```python
from build123d import *

# Parameters (mm, degrees)
F0_W      = 1397
F0_H      = 355.6
F1_DEPTH  = 920.75
F9_W      = 330.2
F9_H      = 330.2
F10_DEPTH = 279.4
F7_W      = 330.2
F7_H      = 330.2
F11_DEPTH = 279.4
F5_W      = 330.2
F5_H      = 330.2
F12_DEPTH = 279.4
F3_W      = 330.2
F3_H      = 330.2
F13_DEPTH = 279.4


with BuildPart() as f1:
    # F0 (on Top) → F1 (new body)
    with BuildSketch(Plane.XY):
        with Locations((698.5, -177.8)):
            Rectangle(F0_W, F0_H)
    extrude(amount=F1_DEPTH)

    # F9 (on face) → F10 (cut)
    with BuildSketch(Plane.XY.offset(920.75)):
        with Locations((190.5, -177.8)):
            Rectangle(F9_W, F9_H)
    extrude(amount=-F10_DEPTH, mode=Mode.SUBTRACT)

    # F7 (on face) → F11 (cut)
    with BuildSketch(Plane.XY.offset(920.75)):
        with Locations((533.4, -177.8)):
            Rectangle(F7_W, F7_H)
    extrude(amount=-F11_DEPTH, mode=Mode.SUBTRACT)

    # F5 (on face) → F12 (cut)
    with BuildSketch(Plane.XY.offset(920.75)):
        with Locations((876.3, -177.8)):
            Rectangle(F5_W, F5_H)
    extrude(amount=-F12_DEPTH, mode=Mode.SUBTRACT)

    # F3 (on face) → F13 (cut)
    with BuildSketch(Plane.XY.offset(920.75)):
        with Locations((1219.2, -177.8)):
            Rectangle(F3_W, F3_H)
    extrude(amount=-F13_DEPTH, mode=Mode.SUBTRACT)

    # F14: F1 across plane


with BuildPart() as f1_1:
    add(f1.part)
    add(f1.part.mirror(Plane.XZ))


solid = f1_1.part
```
Source: CAD feature listing. Evaluate the final solid. Frame: model axes, mm. Round coordinates to 2 decimals unless told otherwise and drop trailing zeros. Loops run counter-clockwise (first coordinate to the right, second up) from the corner with the lowest first, then second, coordinate; pieces in that order, holes last. Notation, with made-up numbers: (-35.75, 28) - (15.25, 28) arc R7 ccw to (15.25, 35) - close; hole circle Ø11 at (21, 53). An arc over 180 degrees is marked (long way). Use CSV: the item, a comma, the result in double quotes.
Q1. Section query B-B, the plane y = 253.5. Output: boundary loops of the cut face in (x, z), then the cut area to 3 significant figures.
Reported:
outline,"(0, 0) - (1397, 0) - (1397, 920.75) - (1384.3, 920.75) - (1384.3, 641.35) - (1054.1, 641.35) - (1054.1, 920.75) - (1041.4, 920.75) - (1041.4, 641.35) - (711.2, 641.35) - (711.2, 920.75) - (698.5, 920.75) - (698.5, 641.35) - (368.3, 641.35) - (368.3, 920.75) - (355.6, 920.75) - (355.6, 641.35) - (25.4, 641.35) - (25.4, 920.75) - (0, 920.75) - close"
area,"917,000 mm^2"
Q2. Mould query, pull axis X, two halves, no side actions, for faces 1 (the flat face through (188, -12.7, 783)), 2 (the flat face through (689, -5, 0)). Classes: pulls with the +X half, pulls with the -X half, needs draft (parallel to the pull), parting line crosses it, or undercut.
Reported:
face 1,"undercut"
face 2,"needs draft"
Q3. Section query C-C, the plane z = 786. Give the number of separate pieces and of enclosed holes in the cut face, then the cut area to 3 significant figures.
Reported:
separate pieces,"1"
enclosed holes,"8"
area,"121,000 mm^2"
Q4. Ray query, line 1 along Y through (x, z) = (384, 755); line 2 along X through (y, z) = (-241, 769); line 3 along Z through (x, y) = (275, 29.5). Return the intervals inside material, ascending.
Reported:
line 1,"-355.6 to -342.9, -12.7 to 12.7, 342.9 to 355.6"
line 2,"0 to 25.4, 355.6 to 368.3, 698.5 to 711.2, 1041.4 to 1054.1, 1384.3 to 1397"
line 3,"0 to 641.35"
Q5. Pin query (flat end, axial travel): pin 1 Ø6 at (x, y) = (622.5, -105) entering from +Z; pin 2 Ø4 at (x, y) = (1197, 119) entering from -Z. Return the tip coordinate at first contact, or that it passes through.
Reported:
pin 1,"z = 641.35"
pin 2,"z = 0"
Q6. Section query A-A, the plane x = 1257. Output: boundary loops of the cut face in (y, z), then the cut area to 3 significant figures.
Reported:
outline,"(-355.6, 0) - (355.6, 0) - (355.6, 920.75) - (342.9, 920.75) - (342.9, 641.35) - (12.7, 641.35) - (12.7, 920.75) - (-12.7, 920.75) - (-12.7, 641.35) - (-342.9, 641.35) - (-342.9, 920.75) - (-355.6, 920.75) - close"
area,"470,000 mm^2"
